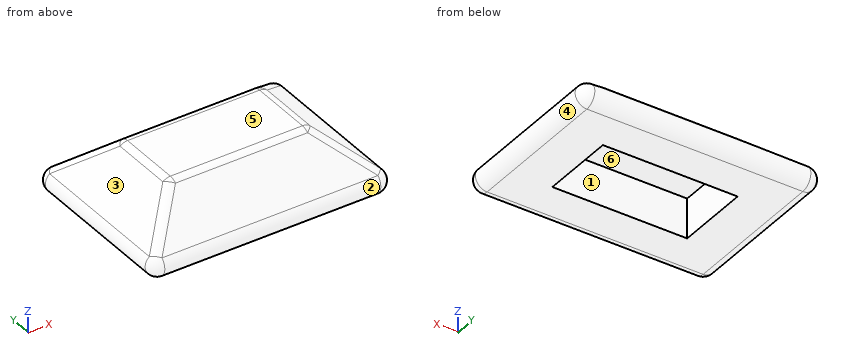
```python
from build123d import *

# Parameters (mm, degrees)
SKETCH_1_W          = 119.8195585
SKETCH_1_H          = 61.146113558
EXTRUDE_1_DEPTH     = 50
DRAFT_8_ANGLE       = 50
FILLET_1_R          = 10
SKETCH_2_W          = 114.826849908
SKETCH_2_H          = 63.442671994
CUT_EXTRUDE_1_DEPTH = 34


with BuildPart() as part:
    # 草图1 → 凸台-拉伸1 (new body)
    with BuildSketch(Plane.XY):
        Rectangle(SKETCH_1_W, SKETCH_1_H)
    extrude(amount=EXTRUDE_1_DEPTH)

    # 拔模8
    draft_8_faces = [part.faces().sort_by_distance(p)[0] for p in [
        (-59.90977925, 0, 25),
        (0, -30.573056779, 25),
        (59.90977925, 0, 25),
        (0, 30.573056779, 25),
    ]]
    draft(draft_8_faces, Plane.XY.offset(50), DRAFT_8_ANGLE)

    # 圆角1
    fillet_1_edges = [part.edges().sort_by_distance(p)[0] for p in [
        (59.90977925, 0, 50),
        (0, 30.573056779, 50),
        (-59.90977925, 0, 50),
        (0, 90.160736408, 0),
        (119.49745888, 0, 0),
        (0, -90.160736408, 0),
        (-119.49745888, 0, 0),
        (0, -30.573056779, 50),
        (-89.703619065, 60.366896593, 25),
        (89.703619065, 60.366896593, 25),
        (89.703619065, -60.366896593, 25),
        (-89.703619065, -60.366896593, 25),
    ]]
    fillet(fillet_1_edges, radius=FILLET_1_R)

    # 草图2 → 切除-拉伸1 (cut)
    with BuildSketch(Plane(origin=(0, 0, 0), x_dir=(-1, 0, 0), z_dir=(0, 0, -1))):
        Rectangle(SKETCH_2_W, SKETCH_2_H)
    extrude(amount=-CUT_EXTRUDE_1_DEPTH, mode=Mode.SUBTRACT)


solid = part.part
```
Geometry check sheet. Reference: the model listing, model coordinates, mm. Face numbers are marked on the shaded views. A direction names the side the tool comes from. Round coordinates to 2 decimals unless told otherwise and drop trailing zeros. Order: outer loops, then holes, each group sorted by start corner. A loop starts at its lowest first (then second) coordinate and runs counter-clockwise, first axis right, second up. Notation, with made-up numbers: M 75.25,41.5 L 120.25,41.5 A8 ccw 120.25,47.5 Z; hole C 20.25,47.25 d8. An arc over 180 degrees is marked long. Write item = value, one per line.
Q1. Section check B-B (x = 38.5). Enter the section's corners in (y, z), plus the area to 3 significant figures.
Answer block:
outline = M -69.11,17.66 A10 ccw -62.69,0 L -31.72,0 L -31.72,34 L 31.72,34 L 31.72,0 L 62.69,0 A10 ccw 69.11,17.66 L 33.36,47.66 A10 ccw 26.93,50 L -26.93,50 A10 ccw -33.36,47.66 Z
area = 3,570 mm^2
Q2. Set-up check for the marked faces 5 and 6: record each of +Z, -Z, +X, -X, +Y, -Y from which the full face is reachable in a straight line by a thin tool's end or side.
Answer block:
face_5 = +Z, +X, -X, +Y, -Y
face_6 = -Z
Q3. Section check C-C (z = 14). Enter the section's corners in (x, y), plus the area to 3 significant figures.
Answer block:
outline = M -101.19,-62.69 A9.17 ccw -92.02,-71.85 L 92.02,-71.85 A9.17 ccw 101.19,-62.69 L 101.19,62.69 A9.17 ccw 92.02,71.85 L -92.02,71.85 A9.17 ccw -101.19,62.69 Z; hole M -57.41,-31.72 L 57.41,-31.72 L 57.41,31.72 L -57.41,31.72 Z
area = 21,700 mm^2
Q4. Release check for a two-part mould opening along X. For the marked faces 1, 2, 3 and 4 record: released by +X, released by -X, zero draft, split by the parting line, or undercut.
Answer block:
face_1 = undercut
face_2 = zero draft
face_3 = released by -X
face_4 = released by +X
Q5. Depth check by flat-ended pin: pin 1 Ø1 at (y, z) = (-37.5, 14) entering from +X; pin 2 Ø3 at (y, z) = (-21, 42) entering from +X; pin 3 Ø8 at (y, z) = (-14.5, 37.5) entering from +X. Enter the tip coordinate at first touch or a pass-through.
Answer block:
pin_1 = 101.39
pin_2 = 71.23
pin_3 = 79.57
Q6. Scan lines: line 1 (Z direction, x = -25.5, y = 12.5); line 2 (X direction, y = -14, z = 19); line 3 (X direction, y = 18, z = 5.5). Record each from-to range of solid material in increasing order.
Answer block:
line_1 = 34 to 50
line_2 = -96.85 to -57.41, 57.41 to 96.85
line_3 = -100.95 to -57.41, 57.41 to 100.95
Q7. Section check A-A (y = 11). Enter the section's corners in (x, z), plus the area to 3 significant figures.
Answer block:
outline = M -98.45,17.66 A10 ccw -92.02,0 L -57.41,0 L -57.41,34 L 57.41,34 L 57.41,0 L 92.02,0 A10 ccw 98.45,17.66 L 62.7,47.66 A10 ccw 56.27,50 L -56.27,50 A10 ccw -62.7,47.66 Z
area = 4,760 mm^2
